Job drawing, mm, ordinate dimensions from the low corner. One solid piece. A direction names the side the tool comes from. Give positions to 0.01 mm unless a question says otherwise; leave off trailing zeros. Order: outer loops, then holes, each group sorted by start corner. A loop starts at its lowest first (then second) coordinate and runs counter-clockwise, first axis right, second up. Notation, with made-up numbers: M -32.5,19.25 L 1.5,19.25 A35 ccw 1.5,58.25 Z; hole C -21.5,24.25 d7. An arc over 180 degrees is marked long. Put each result on its own line as item: value. Start each with the question number.
1) Drill centre lines: line 1 (X direction, y = 58, z = 21.5); line 2 (Y direction, x = 63, z = 24); line 3 (Z direction, x = 137, y = 4.5). Where is each one in solid material? Low to high. Write a range as [from, to].
2) Pin check, flat tips, straight feed: pin 1 (6 mm diameter, centred on x = 527, y = 21, fed in from +Z); pin 2 (1 mm diameter, centred on x = 207, z = 30.5, fed in from +Y); pin 3 (10 mm diameter, centred on x = 172.5, z = 114.5, fed in from -Y). Stop position of each tip, or through.
3) Two-plate mould, pull along X, no slides. Class the marked faces 1, 2 and 3: released by +X, released by -X, zero draft, split by the parting line, or undercut.
4) Cut at B-B (y = 44.5). Write the cut outline in (x, z).
5) Cut at A-A (x = 284). Write the cut outline in (y, z), and give its area (3 significant figures).
6) Cut at D-D (y = 13.5). Write the cut outline in (x, z), and give its area (3 significant figures).
7) Tool access for the marked faces 4 and 5: list every direction of +Z, -Z, +X, -X, +Y, -Y with a clear straight run to the whole face (end or side of a thin tool).
8) Cut at C-C (z = 36). Write the cut outline in (x, y), and give its area (3 significant figures).
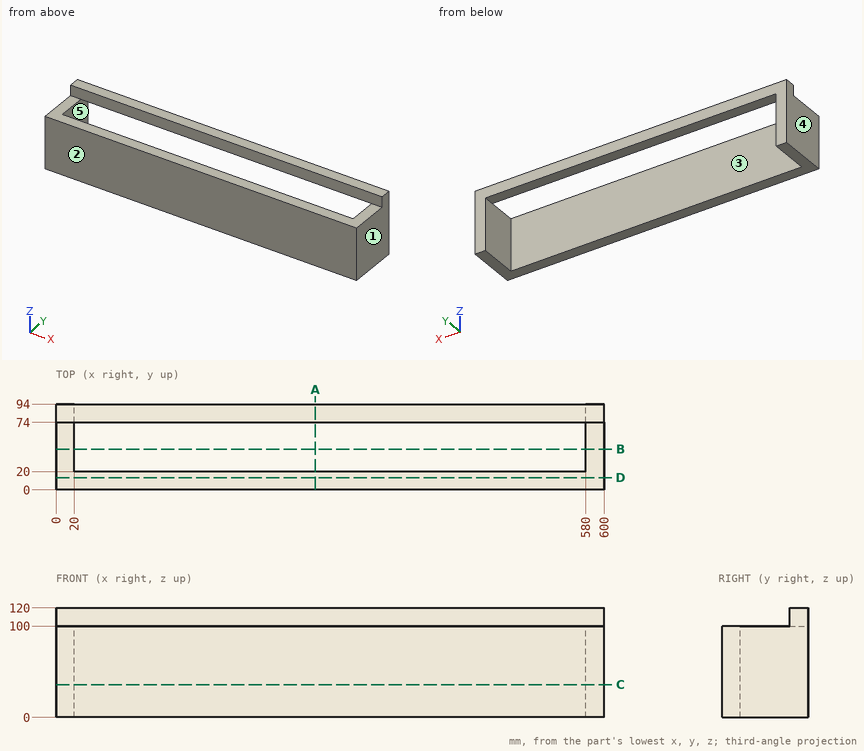
Solution:
1. line 1: [0, 20], [580, 600]
1. line 2: [0, 20]
1. line 3: [0, 100]
2. pin 1: z = 100
2. pin 2: y = 20
2. pin 3: y = 74
3. face 1: released by +X
3. face 2: zero draft
3. face 3: undercut
4. outline: M 0,0 L 20,0 L 20,100 L 0,100 Z; M 580,0 L 600,0 L 600,100 L 580,100 Z
5. outline: M 0,0 L 20,0 L 20,100 L 0,100 Z; M 74,100 L 94,100 L 94,120 L 74,120 Z
5. area: 2,400 mm²
6. outline: M 0,0 L 600,0 L 600,100 L 0,100 Z
6. area: 60,000 mm²
7. face 4: +Z, -Z, -X, +Y, -Y
7. face 5: -Z, +Y
8. outline: M 0,0 L 600,0 L 600,94 L 580,94 L 580,20 L 20,20 L 20,94 L 0,94 Z
8. area: 15,000 mm²
